Part model, mm, in its own coordinate system. Face numbers are marked on the shaded views. A direction names the side the tool comes from. Round coordinates to 2 decimals unless told otherwise and drop trailing zeros. Loops run counter-clockwise (first coordinate to the right, second up) from the corner with the lowest first, then second, coordinate; pieces in that order, holes last. Notation, with made-up numbers: (42, -10) -> (73, -10) arc R20 ccw to (73, 14) -> close; hole circle Ø10 at (68.5, -15.5). An arc over 180 degrees is marked (long way). Use a Markdown table: item, result. Add a question column.
Item 1: Which spindle directions (+Z, -Z, +X, -X, +Y, -Y) get a long thin tool onto all of the face, cutting with end or side? Do the marked faces 1 and 2. Say none if no direction does.
Item 2: Cut at B-B, the plane x = 4.5. List the corners of the cut face in (y, z) (3 decimals).
Item 3: Probe line 1 (X direction, y = -24.4, z = -5.5) (3 decimals); line 2 (X direction, y = 20, z = 6.25) (3 decimals); line 3 (Y direction, x = 2.5, z = 8.75) (3 decimals). List the from-to ranges inside material, lowest first. Write a range as [from, to].
Item 4: Cut at C-C, the plane y = 8. List the corners of the cut face in (x, z) (3 decimals).
Item 5: Flat gauge pins, fed straight in: pin 1 (12.5 mm diameter, centred on x = -6, z = -4.5, fed in from +Y) (3 decimals); pin 2 (5 mm diameter, centred on y = -12, z = 5.5, fed in from -X) (3 decimals); pin 3 (3 mm diameter, centred on x = 3.875, z = -5.5, fed in from -Y). Where does each tip first touch, or does it go through?
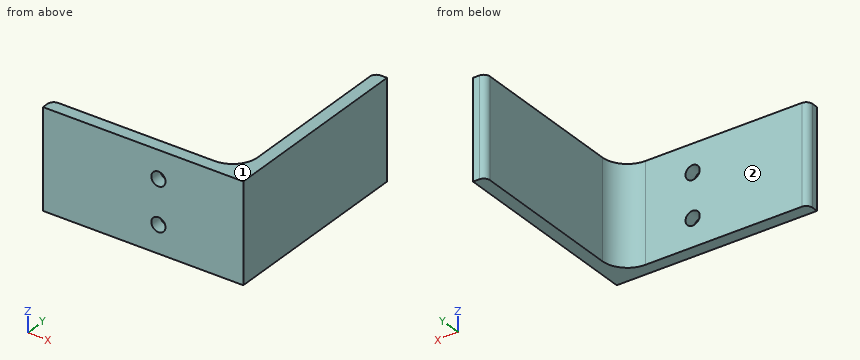
```python
from build123d import *

# Parameters (mm, degrees)
BOSS_EXTRUDE1_DEPTH  = 12.500000019
M3_CLEARANCE_HOLE1_D = 3.6


with BuildPart() as part:
    # Sketch2 → Boss-Extrude1 (new, symmetric)
    with BuildSketch(Plane.XY):
        with BuildLine():
            Line((-25.4, -25.4), (25.4, -25.4))
            Line((25.4, -25.4), (25.4, 25.4))
            Line((25.4, 25.4), (23.8125, 25.4))
            ThreePointArc((23.8125, 25.4), (22.689967985, 24.935032015), (22.225, 23.8125))
            Line((22.225, 23.8125), (22.225, -15.875))
            ThreePointArc((22.225, -15.875), (20.365128061, -20.365128061), (15.875, -22.225))
            Line((15.875, -22.225), (-23.8125, -22.225))
            ThreePointArc((-23.8125, -22.225), (-24.935032015, -22.689967985), (-25.4, -23.8125))
            Line((-25.4, -23.8125), (-25.4, -25.4))
        make_face()
    extrude(amount=BOSS_EXTRUDE1_DEPTH, both=True)

    # M3 Clearance Hole1 (through all)
    with Locations(Plane(origin=(0, -22.225, 0), x_dir=(1, 0, 0), z_dir=(0, 1, 0))):
        with Locations((3.875000124, 5.500000049), (3.875000124, -5.500000049)):
            Hole(M3_CLEARANCE_HOLE1_D / 2)


solid = part.part
```
A:
| question | item | result |
|---|---|---|
| 1 | face 1 | +Z, +X, -X, +Y, -Y |
| 1 | face 2 | +Z, -Z, -X, +Y |
| 2 | outline | (-25.4, -12.5) -> (-22.225, -12.5) -> (-22.225, -7.188) -> (-25.4, -7.188) -> close; (-25.4, -3.812) -> (-22.225, -3.812) -> (-22.225, 3.812) -> (-25.4, 3.812) -> close; (-25.4, 7.188) -> (-22.225, 7.188) -> (-22.225, 12.5) -> (-25.4, 12.5) -> close |
| 3 | line 1 | x = [-25.4, 2.075], [5.675, 25.4] |
| 3 | line 2 | x = [22.225, 25.4] |
| 3 | line 3 | y = [-25.4, -22.225] |
| 4 | outline | (22.225, -12.5) -> (25.4, -12.5) -> (25.4, 12.5) -> (22.225, 12.5) -> close |
| 5 | pin 1 | stops at y = -22.225 |
| 5 | pin 2 | stops at x = 22.225 |
| 5 | pin 3 | passes through |
